Work out the finished part from the listing and answer in its coordinate system (mm). Give positions to 0.01 mm unless a question says otherwise; leave off trailing zeros. Loops run counter-clockwise (first coordinate to the right, second up) from the corner with the lowest first, then second, coordinate; pieces in that order, holes last. Notation, with made-up numbers: M 22,6.25 L 79,6.25 A9 cw 79,13.25 Z; hole C 84.5,67.5 d1. An arc over 180 degrees is marked long. Answer in a Markdown table with one row per item. Add a question column.
from build123d import *

# Parameters (mm, degrees)
SKETCH1_R           = 1.825
BOSS_EXTRUDE1_DEPTH = 1.5
CUT_EXTRUDE1_REACH  = 41.08
SKETCH2_R           = 1
SKETCH2_R_2         = 0.75
SKETCH2_R_3         = 0.5


with BuildPart() as part:
    # Sketch1 → Boss-Extrude1 (new body)
    with BuildSketch(Plane(origin=(0, 0, 0), x_dir=(1, 0, 0), z_dir=(0, 1, 0))):
        with BuildLine():
            Line((-21, 30), (21, 30))
            ThreePointArc((21, 30), (23.828427125, 28.828427125), (25, 26))
            Line((25, 26), (25, -26))
            ThreePointArc((25, -26), (23.828427125, -28.828427125), (21, -30))
            Line((21, -30), (-21, -30))
            ThreePointArc((-21, -30), (-23.828427125, -28.828427125), (-25, -26))
            Line((-25, -26), (-25, 26))
            ThreePointArc((-25, 26), (-23.828427125, 28.828427125), (-21, 30))
        make_face()
        with Locations(Location((-21, 26, 0), (0, 0, 270))):
            Circle(SKETCH1_R, mode=Mode.SUBTRACT)
        with Locations(Location((21, 26, 0), (0, 0, 90))):
            Circle(SKETCH1_R, mode=Mode.SUBTRACT)
        with Locations(Location((21, -26, 0), (0, 0, 270))):
            Circle(SKETCH1_R, mode=Mode.SUBTRACT)
        with Locations(Location((-21, -26, 0), (0, 0, 90))):
            Circle(SKETCH1_R, mode=Mode.SUBTRACT)
    extrude(amount=BOSS_EXTRUDE1_DEPTH)

    # Sketch2 → Cut-Extrude1 (cut, up to next)
    with BuildSketch(Plane(origin=(0, 1.5, 0), x_dir=(1, 0, 0), z_dir=(0, 1, 0)), mode=Mode.PRIVATE) as cut_extrude1_sk1:
        with Locations(Location((-9, 16, 0), (0, 0, 270))):
            Circle(SKETCH2_R)
    cut_extrude1_tool1 = extrude(cut_extrude1_sk1.sketch, amount=-CUT_EXTRUDE1_REACH, mode=Mode.PRIVATE) & part.part
    # Sketch2 → Cut-Extrude1 (cut, up to next)
    with BuildSketch(Plane(origin=(0, 1.5, 0), x_dir=(1, 0, 0), z_dir=(0, 1, 0)), mode=Mode.PRIVATE) as cut_extrude1_sk2:
        with Locations(Location((9, 16, 0), (0, 0, 270))):
            Circle(SKETCH2_R)
    cut_extrude1_tool2 = extrude(cut_extrude1_sk2.sketch, amount=-CUT_EXTRUDE1_REACH, mode=Mode.PRIVATE) & part.part
    # Sketch2 → Cut-Extrude1 (cut, up to next)
    with BuildSketch(Plane(origin=(0, 1.5, 0), x_dir=(1, 0, 0), z_dir=(0, 1, 0)), mode=Mode.PRIVATE) as cut_extrude1_sk3:
        with Locations(Location((-5.25, 12, 0), (0, 0, 270))):
            Circle(SKETCH2_R_2)
    cut_extrude1_tool3 = extrude(cut_extrude1_sk3.sketch, amount=-CUT_EXTRUDE1_REACH, mode=Mode.PRIVATE) & part.part
    # Sketch2 → Cut-Extrude1 (cut, up to next)
    with BuildSketch(Plane(origin=(0, 1.5, 0), x_dir=(1, 0, 0), z_dir=(0, 1, 0)), mode=Mode.PRIVATE) as cut_extrude1_sk4:
        with Locations(Location((0, 12, 0), (0, 0, 270))):
            Circle(SKETCH2_R_2)
    cut_extrude1_tool4 = extrude(cut_extrude1_sk4.sketch, amount=-CUT_EXTRUDE1_REACH, mode=Mode.PRIVATE) & part.part
    # Sketch2 → Cut-Extrude1 (cut, up to next)
    with BuildSketch(Plane(origin=(0, 1.5, 0), x_dir=(1, 0, 0), z_dir=(0, 1, 0)), mode=Mode.PRIVATE) as cut_extrude1_sk5:
        with Locations(Location((5.25, 12, 0), (0, 0, 270))):
            Circle(SKETCH2_R_2)
    cut_extrude1_tool5 = extrude(cut_extrude1_sk5.sketch, amount=-CUT_EXTRUDE1_REACH, mode=Mode.PRIVATE) & part.part
    # Sketch2 → Cut-Extrude1 (cut, up to next)
    with BuildSketch(Plane(origin=(0, 1.5, 0), x_dir=(1, 0, 0), z_dir=(0, 1, 0)), mode=Mode.PRIVATE) as cut_extrude1_sk6:
        with Locations(Location((-15.25, -7.5, 0), (0, 0, 270))):
            Circle(SKETCH2_R)
    cut_extrude1_tool6 = extrude(cut_extrude1_sk6.sketch, amount=-CUT_EXTRUDE1_REACH, mode=Mode.PRIVATE) & part.part
    # Sketch2 → Cut-Extrude1 (cut, up to next)
    with BuildSketch(Plane(origin=(0, 1.5, 0), x_dir=(1, 0, 0), z_dir=(0, 1, 0)), mode=Mode.PRIVATE) as cut_extrude1_sk7:
        with Locations(Location((-5.25, -7.5, 0), (0, 0, 270))):
            Circle(SKETCH2_R)
    cut_extrude1_tool7 = extrude(cut_extrude1_sk7.sketch, amount=-CUT_EXTRUDE1_REACH, mode=Mode.PRIVATE) & part.part
    # Sketch2 → Cut-Extrude1 (cut, up to next)
    with BuildSketch(Plane(origin=(0, 1.5, 0), x_dir=(1, 0, 0), z_dir=(0, 1, 0)), mode=Mode.PRIVATE) as cut_extrude1_sk8:
        with Locations(Location((5.25, -7.5, 0), (0, 0, 270))):
            Circle(SKETCH2_R)
    cut_extrude1_tool8 = extrude(cut_extrude1_sk8.sketch, amount=-CUT_EXTRUDE1_REACH, mode=Mode.PRIVATE) & part.part
    # Sketch2 → Cut-Extrude1 (cut, up to next)
    with BuildSketch(Plane(origin=(0, 1.5, 0), x_dir=(1, 0, 0), z_dir=(0, 1, 0)), mode=Mode.PRIVATE) as cut_extrude1_sk9:
        with Locations(Location((15.25, -7.5, 0), (0, 0, 270))):
            Circle(SKETCH2_R)
    cut_extrude1_tool9 = extrude(cut_extrude1_sk9.sketch, amount=-CUT_EXTRUDE1_REACH, mode=Mode.PRIVATE) & part.part
    # Sketch2 → Cut-Extrude1 (cut, up to next)
    with BuildSketch(Plane(origin=(0, 1.5, 0), x_dir=(1, 0, 0), z_dir=(0, 1, 0)), mode=Mode.PRIVATE) as cut_extrude1_sk10:
        with Locations(Location((-18, 9, 0), (0, 0, 270))):
            Circle(SKETCH2_R_3)
    cut_extrude1_tool10 = extrude(cut_extrude1_sk10.sketch, amount=-CUT_EXTRUDE1_REACH, mode=Mode.PRIVATE) & part.part
    # Sketch2 → Cut-Extrude1 (cut, up to next)
    with BuildSketch(Plane(origin=(0, 1.5, 0), x_dir=(1, 0, 0), z_dir=(0, 1, 0)), mode=Mode.PRIVATE) as cut_extrude1_sk11:
        with Locations(Location((-18, 6.5, 0), (0, 0, 270))):
            Circle(SKETCH2_R_3)
    cut_extrude1_tool11 = extrude(cut_extrude1_sk11.sketch, amount=-CUT_EXTRUDE1_REACH, mode=Mode.PRIVATE) & part.part
    add(cut_extrude1_tool1.solids().sort_by_distance((-9, 1.5, -16))[0], mode=Mode.SUBTRACT)
    add(cut_extrude1_tool2.solids().sort_by_distance((9, 1.5, -16))[0], mode=Mode.SUBTRACT)
    add(cut_extrude1_tool3.solids().sort_by_distance((-5.25, 1.5, -12))[0], mode=Mode.SUBTRACT)
    add(cut_extrude1_tool4.solids().sort_by_distance((0, 1.5, -12))[0], mode=Mode.SUBTRACT)
    add(cut_extrude1_tool5.solids().sort_by_distance((5.25, 1.5, -12))[0], mode=Mode.SUBTRACT)
    add(cut_extrude1_tool6.solids().sort_by_distance((-15.25, 1.5, 7.5))[0], mode=Mode.SUBTRACT)
    add(cut_extrude1_tool7.solids().sort_by_distance((-5.25, 1.5, 7.5))[0], mode=Mode.SUBTRACT)
    add(cut_extrude1_tool8.solids().sort_by_distance((5.25, 1.5, 7.5))[0], mode=Mode.SUBTRACT)
    add(cut_extrude1_tool9.solids().sort_by_distance((15.25, 1.5, 7.5))[0], mode=Mode.SUBTRACT)
    add(cut_extrude1_tool10.solids().sort_by_distance((-18, 1.5, -9))[0], mode=Mode.SUBTRACT)
    add(cut_extrude1_tool11.solids().sort_by_distance((-18, 1.5, -6.5))[0], mode=Mode.SUBTRACT)


solid = part.part
(1) Consider line 1 along X through (y, z) = (0.75, 26) (3 decimals); line 2 along X through (y, z) = (0.4, 7.5); line 3 along X through (y, z) = (0.6, -12). Determine where each line is inside the solid, lowest interval first. Write a range as from..to.
(2) Section C-C, the plane y = 1.15 is taken. State how many separate pieces and enclosed holes the cut face has, and give its area (3 significant figures).
(3) The mould has two halves that part along X. Classify faces 1 (the face through (0, 1, 30)), 2 (the face through (23.797, 0.74, -28.859)), 3 (the face through (-19.22, 0.74, 26.4)): pulls with the +X half, pulls with the -X half, needs draft (parallel to the pull), parting line crosses it, or undercut.
(4) Section A-A, the plane x = -5.25 is taken. Determine the outline of the cut face in (y, z), and give its area (4 significant figures).
(5) Section B-B, the plane z = -16 is taken. Determine the outline of the cut face in (x, y).
(6) Each of these flat-tipped pins is pushed along its axis until it touches: P1, Ø1.8, axis at x = -15.25, z = 7.5, coming from the -Y side; P2, Ø3, axis at x = 9, z = -16, coming from the +Y side. Where does it stop, or does it pass through?
Numbers:
| question | item | result |
|---|---|---|
| 1 | line 1 | x = -25..-22.825, -19.175..19.175, 22.825..25 |
| 1 | line 2 | x = -25..-16.25, -14.25..-6.25, -4.25..4.25, 6.25..14.25, 16.25..25 |
| 1 | line 3 | x = -25..-6, -4.5..-0.75, 0.75..4.5, 6..25 |
| 2 | separate pieces | 1 |
| 2 | enclosed holes | 15 |
| 2 | area | 2,920 mm² |
| 3 | face 1 | needs draft |
| 3 | face 2 | pulls with the +X half |
| 3 | face 3 | undercut |
| 4 | outline | M 0,-30 L 1.5,-30 L 1.5,-12.75 L 0,-12.75 Z; M 0,-11.25 L 1.5,-11.25 L 1.5,6.5 L 0,6.5 Z; M 0,8.5 L 1.5,8.5 L 1.5,30 L 0,30 Z |
| 4 | area | 84.75 mm² |
| 5 | outline | M -25,0 L -10,0 L -10,1.5 L -25,1.5 Z; M -8,0 L 8,0 L 8,1.5 L -8,1.5 Z; M 10,0 L 25,0 L 25,1.5 L 10,1.5 Z |
| 6 | P1 | passes through |
| 6 | P2 | stops at y = 1.5 |
